Check sheet for the drawn part. Datum: minimum x, y, z corner. Units: mm. A direction names the side the tool comes from. Give positions to 0.01 mm unless a question says otherwise; leave off trailing zeros. Write each loop counter-clockwise with the first axis right and the second up, starting at its lowest first coordinate (ties: lowest second). Pieces come first, ordered by that corner, then holes. Notation, with made-up numbers: (-33.75, -37.75) - (-3.75, -37.75) arc R10 ccw to (-3.75, -18.75) - close; hole circle Ø2 at (-33, 64.25). An arc over 180 degrees is marked (long way). Answer as a JSON object with one key per item and string values. Group by question number.
Item 1: Sectioned sample at D-D, the plane y = 16. Record the boundary of the cut face in (x, z) (1 decimal).
Item 2: Tool access check on the marked faces 1 and 2. Record the directions out of +Z, -Z, +X, -X, +Y, -Y that give a thin tool (end or side, any length) a straight path to the whole face; none if there is none.
Item 3: Scan lines: line 1 along Y through (x, z) = (38, 10.25); line 2 along X through (y, z) = (26, 9.5); line 3 along Y through (x, z) = (45, 3.5). Record each from-to range of solid material in increasing order. Write a range as [from, to].
Item 4: Go/stop test with flat-tipped pins: pin 1 (6 mm diameter, centred on y = 30.5, z = 8, fed in from +X); pin 2 (5 mm diameter, centred on x = 29.5, z = 9.5, fed in from -Y); pin 3 (3 mm diameter, centred on x = 38.5, z = 6.5, fed in from -Y). Record where each tip stops, or that it passes through.
Item 5: Sectioned sample at A-A, the plane x = 38.1. Record the boundary of the cut face in (y, z), and give its area (3 significant figures).
Item 6: Sectioned sample at B-B, the plane z = 5.75. Record the boundary of the cut face in (x, y) (1 decimal).
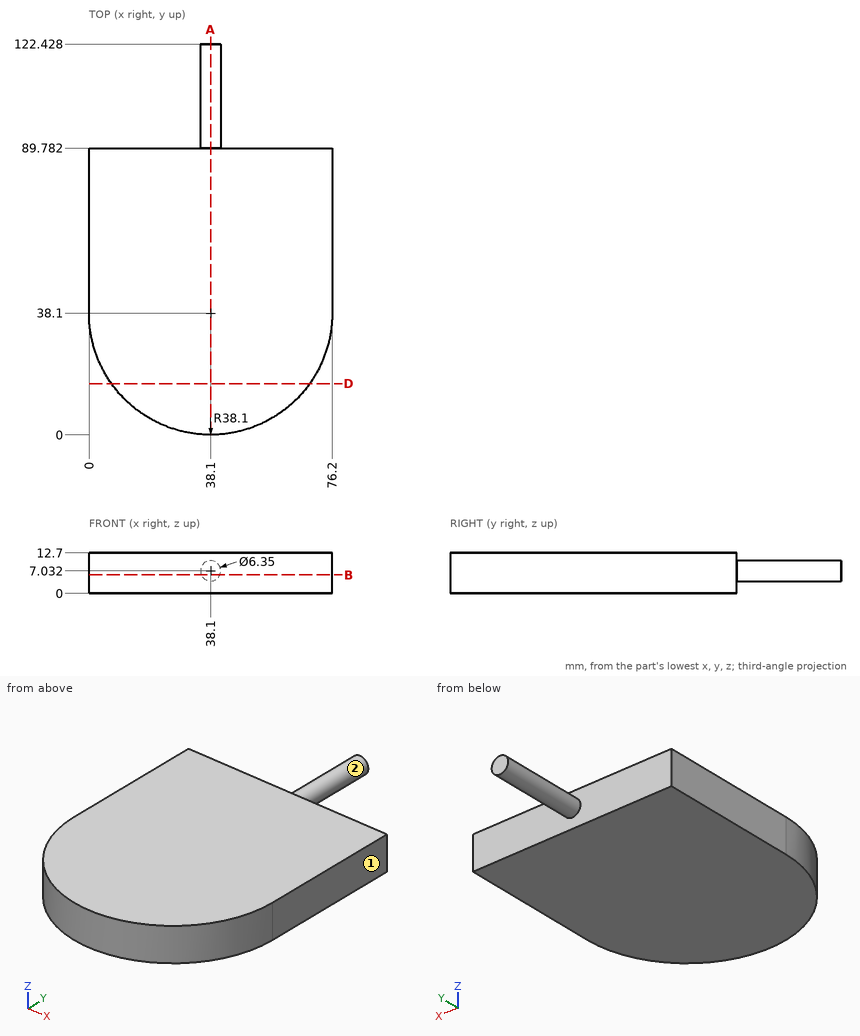
Geometry check:
{
 "1": {"outline": "(7.1, 0) - (69.1, 0) - (69.1, 12.7) - (7.1, 12.7) - close"},
 "2": {"face 1": "+Z, -Z, +X, +Y, -Y", "face 2": "+Y"},
 "3": {"line 1": "[0, 89.78]", "line 2": "[1.97, 74.23]", "line 3": "[0.63, 89.78]"},
 "4": {"pin 1": "x = 75.92", "pin 2": "y = 0.49", "pin 3": "y = 0"},
 "5": {"outline": "(0, 0) - (89.78, 0) - (89.78, 3.86) - (122.43, 3.86) - (122.43, 10.21) - (89.78, 10.21) - (89.78, 12.7) - (0, 12.7) - close", "area": "1,350 mm^2"},
 "6": {"outline": "(0, 38.1) arc R38.1 ccw to (76.2, 38.1) - (76.2, 89.8) - (41, 89.8) - (41, 122.4) - (35.2, 122.4) - (35.2, 89.8) - (0, 89.8) - close"}
}
